from build123d import *

# Parameters (mm, degrees)
F0_R     = 3
F0_R_2   = 3.009085
F2_DEPTH = 4
F1_R     = 0.25
F3_DEPTH = 1


with BuildPart() as f2:
    # F0 (on Top) → F2 (new body)
    with BuildSketch(Plane.XY):
        with BuildLine():
            ThreePointArc((-2.943287, 46.660864), (-0.966878, 0.938237), (-46.69002, 2.902697))
            ThreePointArc((-46.69002, 2.902697), (-53.115015, 3.104241), (-52.884477, -3.319779))
            ThreePointArc((-52.884477, -3.319779), (-31.69787, -12.786126), (-8.831983, -8.831983))
            ThreePointArc((-8.831983, -8.831983), (-12.786126, -31.69787), (-3.319779, -52.884477))
            ThreePointArc((-3.319779, -52.884477), (3.104241, -53.115015), (2.902697, -46.69002))
            ThreePointArc((2.902697, -46.69002), (0.938286, -0.966912), (46.660878, -2.943288))
            ThreePointArc((46.660878, -2.943288), (53.085559, -3.145237), (52.85609, 3.27852))
            ThreePointArc((52.85609, 3.27852), (31.667127, 12.75029), (8.796713, 8.796713))
            ThreePointArc((8.796713, 8.796713), (12.75029, 31.667127), (3.27852, 52.85609))
            ThreePointArc((3.27852, 52.85609), (-3.145192, 53.085499), (-2.943287, 46.660864))
        make_face()
        with BuildLine():
            ThreePointArc((-3.907323, -5.886159), (-8.65465, -26.588997), (0.708341, -45.654123))
            ThreePointArc((0.708341, -45.654123), (-2.997064, -46.775303), (-4.382365, -50.390274))
            ThreePointArc((-4.382365, -50.390274), (-12.181233, -30.319052), (-8.159824, -9.164748))
            ThreePointArc((-8.159824, -9.164748), (-7.916828, -8.690968), (-7.667397, -8.220543))
            ThreePointArc((-7.667397, -8.220543), (-5.754898, -7.105639), (-3.907323, -5.886159))
        make_face(mode=Mode.SUBTRACT)
        with BuildLine():
            ThreePointArc((-50.390274, -4.382365), (-46.775303, -2.997064), (-45.654123, 0.708341))
            ThreePointArc((-45.654123, 0.708341), (-26.589057, -8.654679), (-5.88624, -3.907439))
            ThreePointArc((-5.88624, -3.907439), (-7.105676, -5.754958), (-8.220543, -7.667397))
            ThreePointArc((-8.220543, -7.667397), (-8.690968, -7.916828), (-9.164748, -8.159824))
            ThreePointArc((-9.164748, -8.159824), (-30.319052, -12.181233), (-50.390274, -4.382365))
        make_face(mode=Mode.SUBTRACT)
        with BuildLine():
            ThreePointArc((-6.954048, -6.954048), (-5.537825, -4.72203), (-3.973892, -2.590902))
            ThreePointArc((-3.973892, -2.590902), (-0.470244, 0.435462), (2.556183, 3.939056))
            ThreePointArc((2.556183, 3.939056), (4.687049, 5.502753), (6.918778, 6.918778))
            ThreePointArc((6.918778, 6.918778), (5.502695, 4.686965), (3.93893, 2.556023))
            ThreePointArc((3.93893, 2.556023), (0.435502, -0.47028), (-2.590738, -3.973763))
            ThreePointArc((-2.590738, -3.973763), (-4.721944, -5.537766), (-6.954048, -6.954048))
        make_face(mode=Mode.SUBTRACT)
        with Locations((0, -49.996732)):
            Circle(F0_R, mode=Mode.SUBTRACT)
        with Locations((49.967591, -0.040591)):
            Circle(F0_R, mode=Mode.SUBTRACT)
        with Locations((-49.996732, 0)):
            Circle(F0_R_2, mode=Mode.SUBTRACT)
        with Locations((-0.040589, 49.967576)):
            Circle(F0_R, mode=Mode.SUBTRACT)
        with BuildLine():
            ThreePointArc((50.362121, 4.341686), (46.746855, 2.957219), (45.624813, -0.7479))
            ThreePointArc((45.624813, -0.7479), (26.55794, 8.619893), (5.851302, 3.872643))
            ThreePointArc((5.851302, 3.872643), (7.070559, 5.719934), (8.185273, 7.632127))
            ThreePointArc((8.185273, 7.632127), (29.757679, 12.190586), (50.362121, 4.341686))
        make_face(mode=Mode.SUBTRACT)
        with BuildLine():
            ThreePointArc((3.872754, 5.85138), (8.619916, 26.557989), (-0.7479, 45.624799))
            ThreePointArc((-0.7479, 45.624799), (2.957225, 46.746845), (4.341686, 50.362121))
            ThreePointArc((4.341686, 50.362121), (12.190586, 29.757679), (7.632127, 8.185273))
            ThreePointArc((7.632127, 8.185273), (5.719991, 7.070594), (3.872754, 5.85138))
        make_face(mode=Mode.SUBTRACT)
    extrude(amount=F2_DEPTH)

    # F1 (on Top) → F3 (join)
    with BuildSketch(Plane.XY):
        with BuildLine():
            ThreePointArc((-10.960155, 0.353553), (-12.374369, 0.353553), (-12.374369, -1.06066))
            Line((-12.374369, -1.06066), (-6.717514, -6.717514))
            Line((-6.717514, -6.717514), (-1.06066, -12.374369))
            ThreePointArc((-1.06066, -12.374369), (0.353553, -12.374369), (0.353553, -10.960155))
            Line((0.353553, -10.960155), (-5.303301, -5.303301))
            Line((-5.303301, -5.303301), (-10.960155, 0.353553))
        make_face()
        with Locations((-0.353553, -11.667262)):
            Circle(F1_R, mode=Mode.SUBTRACT)
        with Locations((-11.667262, -0.353553)):
            Circle(F1_R, mode=Mode.SUBTRACT)
        with BuildLine():
            ThreePointArc((12.374369, 1.06066), (13.788582, 1.06066), (13.788582, 2.474874))
            Line((13.788582, 2.474874), (8.131728, 8.131728))
            Line((8.131728, 8.131728), (6.717514, 6.717514))
            Line((6.717514, 6.717514), (12.374369, 1.06066))
        make_face()
        with Locations((13.081475, 1.767767)):
            Circle(F1_R, mode=Mode.SUBTRACT)
        with BuildLine():
            Line((6.717514, 6.717514), (8.131728, 8.131728))
            Line((8.131728, 8.131728), (2.474874, 13.788582))
            ThreePointArc((2.474874, 13.788582), (1.06066, 13.788582), (1.06066, 12.374369))
            Line((1.06066, 12.374369), (6.717514, 6.717514))
        make_face()
        with Locations((1.767767, 13.081475)):
            Circle(F1_R, mode=Mode.SUBTRACT)
    extrude(amount=F3_DEPTH)


solid = f2.part
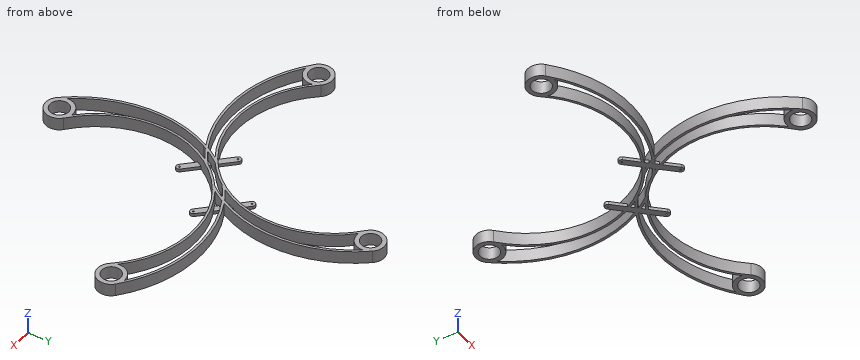
For this review, take the finished solid that the model builds, in its own axes (mm). Give positions to 0.01 mm unless a question says otherwise; leave off trailing zeros. Order: outer loops, then holes, each group sorted by start corner. A loop starts at its lowest first (then second) coordinate and runs counter-clockwise, first axis right, second up. Notation, with made-up numbers: M 18,55.5 L 70,55.5 A19 ccw 70,73.5 Z; hole C -1,-4 d4. An arc over 180 degrees is marked long. Answer in a Markdown table with one row per item. Add a question column.
(1) Consider section C-C on z = 2.1. Give the number of separate pieces and of enclosed holes in the cut face, and give its area (3 significant figures).
(2) Wall thickness on probe 1 along Y at (x, z) = (-3.5, 2.05); probe 2 along Y at (x, z) = (23.5, 0.65); probe 3 along X at (y, z) = (17.5, 3.4): over which ranges is each line inside the solid? List them lowest first. Write a range as [from, to].
(3) Consider section A-A on x = -39.5. State the section outline as (y, z) points.
(4) For pin 1 (1 mm diameter, centred on x = 16, z = 2, fed in from +Y) (3 decimals); pin 2 (1.3 mm diameter, centred on x = 6.5, y = 8.5, fed in from +Z); pin 3 (1 mm diameter, centred on y = -29.5, z = 1, fed in from +X), all flat-tipped, find the tip position at first contact; note any pin that passes through.
(5) Consider section B-B on y = -30.5. State the section outline as (x, z) points, and give its area (3 significant figures).
Evaluation:
| question | item | result |
|---|---|---|
| 1 | separate pieces | 1 |
| 1 | enclosed holes | 9 |
| 1 | area | 425 mm^2 |
| 2 | probe 1 | y = [-52.68, -47.33], [-40.59, -39.29], [-6.57, -4.67], [-2.23, -1.33], [47.25, 52.69] |
| 2 | probe 2 | y = [8.12, 8.83], [12.18, 12.93] |
| 2 | probe 3 | x = [7.65, 8.37], [11.21, 11.98] |
| 3 | outline | M -11,0 L -10.21,0 L -10.21,4 L -11,4 Z; M -4.2,0 L -3.37,0 L -3.37,4 L -4.2,4 Z |
| 4 | pin 1 | stops at y = 11.725 |
| 4 | pin 2 | stops at z = 1 |
| 4 | pin 3 | stops at x = -7.34 |
| 5 | outline | M -12.92,0 L -12.16,0 L -12.16,4 L -12.92,4 Z; M -7.95,0 L -7.22,0 L -7.22,4 L -7.95,4 Z |
| 5 | area | 5.93 mm^2 |
